The model under review builds one solid part; all positions refer to its coordinate system, in mm. Face numbers are marked on the shaded views. A direction names the side the tool comes from. Give positions to 0.01 mm unless a question says otherwise; leave off trailing zeros. Write each loop counter-clockwise with the first axis right and the second up, starting at its lowest first coordinate (ties: lowest second). Pieces come first, ordered by that corner, then holes. Notation, with made-up numbers: M -18.75,83 L -12.75,83 A36 ccw -12.75,119 Z; hole C 20.25,66.5 d6. An arc over 180 degrees is marked long. Write each question's results on one line, items separated by ' | '. Start each with the question number.
from build123d import *

# Parameters (mm, degrees)
BOSS_EXTRUDE1_DEPTH = 18
BOSS_EXTRUDE2_DEPTH = 35
CUT_EXTRUDE1_REACH  = 81.517
SKETCH2_R           = 4


with BuildPart() as part:
    # Sketch1 → Boss-Extrude1 (new, symmetric)
    with BuildSketch(Plane(origin=(0, 0, 0), x_dir=(1, 0, 0), z_dir=(0, 1, 0))):
        with BuildLine():
            Line((0, -32), (0, -57))
            Line((0, -57), (-31.500486732, -57))
            Line((-31.500486732, -57), (-31.500486732, -30.362311102))
            Line((-31.500486732, -30.362311102), (-36, -25))
            Line((-36, -25), (-43, -25))
            Line((-43, -25), (-43, 25))
            Line((-43, 25), (-36, 25))
            Line((-36, 25), (-31.500486732, 30.362311102))
            Line((-31.500486732, 30.362311102), (-31.500486732, 57))
            Line((-31.500486732, 57), (0, 57))
            Line((0, 57), (0, 32))
            ThreePointArc((0, 32), (-32, 0), (0, -32))
        make_face()
    extrude(amount=BOSS_EXTRUDE1_DEPTH, both=True)

    # Sketch1_3 → Boss-Extrude2 (add, symmetric)
    with BuildSketch(Plane(origin=(0, 0, 0), x_dir=(1, 0, 0), z_dir=(0, 1, 0))):
        with BuildLine():
            ThreePointArc((0, -32), (-32, 0), (0, 32))
            Line((0, 32), (0, 26.5))
            ThreePointArc((0, 26.5), (-26.5, 0), (0, -26.5))
            Line((0, -26.5), (0, -32))
        make_face()
    extrude(amount=BOSS_EXTRUDE2_DEPTH, both=True)

    # Sketch2 → Cut-Extrude1 (cut, up to next)
    with BuildSketch(Plane(origin=(0, 0, 0), x_dir=(0, 0, -1), z_dir=(1, 0, 0)), mode=Mode.PRIVATE) as cut_extrude1_sk1:
        with Locations((-45, 0)):
            Circle(SKETCH2_R)
    cut_extrude1_tool1 = extrude(cut_extrude1_sk1.sketch, amount=-CUT_EXTRUDE1_REACH, mode=Mode.PRIVATE) & part.part
    cut_extrude1 = cut_extrude1_tool1.solids().sort_by_distance((0, 0, 45))[0]
    add(cut_extrude1, mode=Mode.SUBTRACT)

    # Mirror1: Cut-Extrude1 across plane
    add(cut_extrude1.mirror(Plane.XY), mode=Mode.SUBTRACT)


solid = part.part
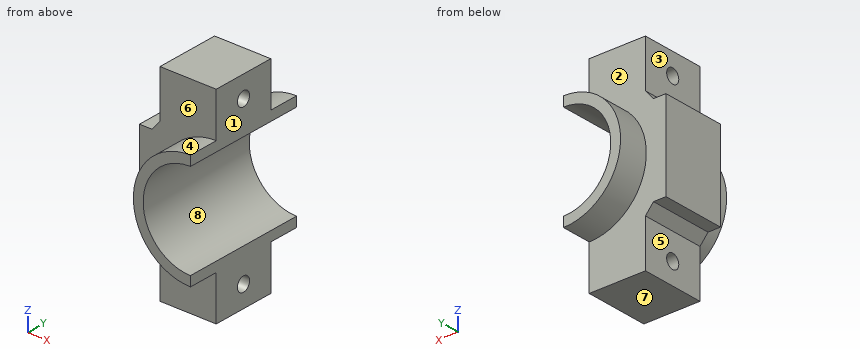
(1) Add section A-A (y = 0). State the section outline as (x, z) points, then the cut area to 3 significant figures.
(2) Add section C-C (z = 45). State the section outline as (x, y) points.
(3) Add section D-D (y = -16). State the section outline as (x, z) points.
(4) Wall thickness on L1, parallel to Y at x = -24.5, z = -45; L2, parallel to Y at x = -37, z = 18; L3, parallel to Z at x = -11.5, y = -2.5: over which ranges is each line inside the solid? List them lowest first.
(5) Clearance check with flat-ended pins moving along their axes: P1, Ø9, axis at y = 0, z = -45, coming from the +X side; P2, Ø1.5, axis at x = -12, z = -22, coming from the -Y side; P3, Ø2, axis at x = -38, y = 6, coming from the +Z side; P4, Ø5.5, axis at x = -39.5, y = 6, coming from the -Z side. State where each tip first meets the part, or that it passes through.
(6) Draft analysis for pull direction Z (two halves, no side actions). For the marked faces 6, 7 and 8, state which applies: pulls with the +Z half, pulls with the -Z half, needs draft (parallel to the pull), parting line crosses it, or undercut.
(7) Machinability: for the marked faces 1, 2, 3, 4 and 5, which of the approach directions +Z, -Z, +X, -X, +Y, -Y give a long, thin tool a straight path to every point of the face, cutting with its end or side? Answer none if there is none.
(8) Add section B-B (x = -20). State the section outline as (y, z) points.
Calculated:
1) outline: M -43,-25 L -36,-25 L -31.5,-30.36 L -31.5,-41 L 0,-41 L 0,-26.5 A26.5 cw 0,26.5 L 0,41 L -31.5,41 L -31.5,30.36 L -36,25 L -43,25 Z; M -31.5,-57 L 0,-57 L 0,-49 L -31.5,-49 Z; M -31.5,49 L 0,49 L 0,57 L -31.5,57 Z | area: 2,580 mm²
2) outline: M -31.5,-18 L 0,-18 L 0,-4 L -31.5,-4 Z; M -31.5,4 L 0,4 L 0,18 L -31.5,18 Z
3) outline: M -43,-25 L -36,-25 L -31.5,-30.36 L -31.5,-57 L 0,-57 L 0,-26.5 A26.5 cw 0,26.5 L 0,57 L -31.5,57 L -31.5,30.36 L -36,25 L -43,25 Z
4) L1: y = -18 to -4, 4 to 18 | L2: y = -18 to 18 | L3: z = -57 to -48.12, -41.88 to -23.87, 23.87 to 41.88, 48.12 to 57
5) P1: stops at x = 0 | P2: passes through | P3: stops at z = 25 | P4: stops at z = -25
6) face 6: needs draft | face 7: pulls with the -Z half | face 8: undercut
7) face 1: +Z, -Z, +X, +Y, -Y | face 2: -X, +Y | face 3: +Z, -X, +Y, -Y | face 4: -X, -Y | face 5: -Z, -X, +Y, -Y
8) outline: M -35,-24.98 L -18,-24.98 L -18,-57 L 18,-57 L 18,-24.98 L 35,-24.98 L 35,-17.39 L -35,-17.39 Z; M -35,17.39 L 35,17.39 L 35,24.98 L 18,24.98 L 18,57 L -18,57 L -18,24.98 L -35,24.98 Z; hole C 0,-45 d8; hole C 0,45 d8
